Build history of the part. All positions in model axes, mm. Face numbers are marked on the shaded views. Round coordinates to 2 decimals unless told otherwise and drop trailing zeros. Order: outer loops, then holes, each group sorted by start corner. A loop starts at its lowest first (then second) coordinate and runs counter-clockwise, first axis right, second up. Notation, with made-up numbers: (12.25, 1) - (71.25, 1) arc R32 cw to (71.25, 35) - close; hole circle Ø4 at (-14.75, 20.5). An arc over 180 degrees is marked (long way). Write each question's results on one line, items separated by ' | '. Start each with the question number.
```python
from build123d import *

# Parameters (mm, degrees)
F1_R     = 21.7223344902
F2_DEPTH = 101.6
F4_DEPTH = 99.02421
F3_R     = 6.1579906
F3_R_2   = 5.385299851
F5_DEPTH = 62.76523


# Not quite as in the source:
# - a feature names something its author has since deleted; it is built from what else it names


with BuildPart() as f2:
    # F1 (on Top) → F2 (new body)
    with BuildSketch(Plane.XY):
        Circle(F1_R)
    extrude(amount=F2_DEPTH)

    # F3 (on face) → F4 (join)
    with BuildSketch(Plane.XY.offset(101.6)):
        with BuildLine():
            ThreePointArc((6.3684736853, -20.7678202666), (11.9405298036, -18.1461721505), (16.5529894413, -14.0662132879))
            ThreePointArc((16.5529894413, -14.0662132879), (8.5555496891, -13.0019756287), (6.3684736853, -20.7678202666))
        make_face()
    extrude(amount=-F4_DEPTH)

    # F3 (on face) → F5 (join)
    with BuildSketch(Plane.XY.offset(101.6)):
        with Locations((11.9405298036, -18.1461721505)):
            Circle(F3_R)
        with Locations((-10.6482523042, 18.933423847)):
            Circle(F3_R_2)
    extrude(amount=-F5_DEPTH)


solid = f2.part
```
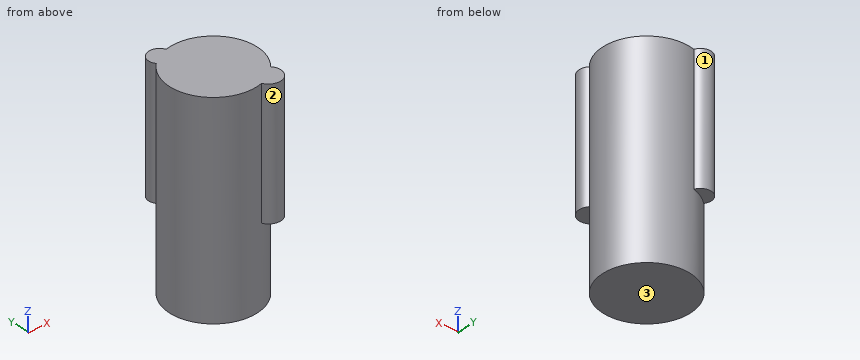
1. Flat gauge pins, fed straight in: pin 1 Ø1.5 at (x, z) = (-2, 56.5) entering from +Y; pin 2 Ø5 at (x, z) = (-3, 41.5) entering from -Y; pin 3 Ø10 at (y, z) = (10.5, 89) entering from +X. Where does each tip first touch, or does it go through?
2. Mould opens along Y. For the marked faces 1, 2 and 3 say: pulls with the +Y half, pulls with the -Y half, needs draft (parallel to the pull), parting line crosses it, or undercut.
3. Cut at B-B (x = 0). List the corners of the cut face in (y, z), plus the area to 3 significant figures.
4. Cut at D-D (x = 9). List the corners of the cut face in (y, z).
5. Cut at A-A (z = 24.5). List the corners of the cut face in (x, y), plus the area to 3 significant figures.
6. Wall check: line 1 (Z direction, x = 14, y = -17.5); line 2 (Y direction, x = 17, z = 44.5); line 3 (Y direction, x = -0.5, z = 37.5). Give the ranges that are in metal, low to high. Write a range as from..to.
7. Cut at C-C (y = -9.5). List the corners of the cut face in (x, z), plus the area to 3 significant figures.
A:
1) pin 1: stops at y = 21.69 | pin 2: stops at y = -21.72 | pin 3: stops at x = 21.01
2) face 1: undercut | face 2: undercut | face 3: needs draft
3) outline: (-21.72, 0) - (21.72, 0) - (21.72, 101.6) - (-21.72, 101.6) - close | area: 4,410 mm^2
4) outline: (-23.56, 38.83) - (-19.77, 38.83) - (-19.77, 0) - (19.77, 0) - (19.77, 101.6) - (-23.56, 101.6) - close
5) outline: circle Ø43.44 at (0, 0) | area: 1,480 mm^2
6) line 1: z = 38.83..101.6 | line 2: y = -21.66..-14.64, -13.52..13.52 | line 3: y = -21.72..21.72
7) outline: (-19.53, 0) - (19.53, 0) - (19.53, 101.6) - (-19.53, 101.6) - close | area: 3,970 mm^2
